from build123d import *

# Parameters (mm, degrees)
CROQUIS1_R              = 25
SALIENTE_EXTRUIR1_DEPTH = 50
CORTAR_EXTRUIR1_REACH   = 102
CROQUIS2_W              = 40
CROQUIS2_H              = 100
CROQUIS3_R              = 25
SALIENTE_EXTRUIR2_DEPTH = 20


with BuildPart() as part:
    # Croquis1 → Saliente-Extruir1 (new body, symmetric)
    with BuildSketch(Plane.XY):
        with BuildLine():
            Line((-50, 0), (50, 0))
            Line((50, 0), (50, 100))
            ThreePointArc((50, 100), (0, 150), (-50, 100))
            Line((-50, 100), (-50, 0))
        make_face()
        with Locations((0, 100)):
            Circle(CROQUIS1_R, mode=Mode.SUBTRACT)
    extrude(amount=SALIENTE_EXTRUIR1_DEPTH, both=True)

    # Croquis2 → Cortar-Extruir1 (cut, up to next)
    with BuildSketch(Plane(origin=(50, 0, 0), x_dir=(0, 0, -1), z_dir=(1, 0, 0)), mode=Mode.PRIVATE) as cortar_extruir1_sk1:
        with Locations((0, 100)):
            Rectangle(CROQUIS2_W, CROQUIS2_H)
    cortar_extruir1_tool1 = extrude(cortar_extruir1_sk1.sketch, amount=-CORTAR_EXTRUIR1_REACH, mode=Mode.PRIVATE) & part.part
    add(cortar_extruir1_tool1.solids().sort_by_distance((50, 100, 0))[0], mode=Mode.SUBTRACT)

    # Croquis3 → Saliente-Extruir2 (add, symmetric)
    with BuildSketch(Plane(origin=(0, 0, 0), x_dir=(0, 0, -1), z_dir=(1, 0, 0))):
        with BuildLine():
            Line((-50, 0), (-50, -150))
            ThreePointArc((-50, -150), (0, -200), (50, -150))
            Line((50, -150), (50, 0))
            Line((50, 0), (-50, 0))
        make_face()
        with Locations((0, -150)):
            Circle(CROQUIS3_R, mode=Mode.SUBTRACT)
    extrude(amount=SALIENTE_EXTRUIR2_DEPTH, both=True)


solid = part.part
Geometry check sheet. Reference: the model listing, model coordinates, mm. A direction names the side the tool comes from. Give positions to 0.01 mm unless a question says otherwise; leave off trailing zeros. Order: outer loops, then holes, each group sorted by start corner. A loop starts at its lowest first (then second) coordinate and runs counter-clockwise, first axis right, second up.
1. Scan lines: line 1 (X direction, y = 100, z = -35); line 2 (X direction, y = -62.5, z = -27); line 3 (Y direction, x = 0, z = -34). Record each from-to range of solid material in increasing order.
Completed:
line 1: x = -50 to -25, 25 to 50
line 2: x = -20 to 20
line 3: y = -186.66 to 75, 125 to 150
2. Sectioned sample at B-B (z = 3). Record the boundary of the cut face in (x, y), then the cut area to 3 significant figures.
Completed:
outline: (-50, 0) - (-20, 0) - (-20, -125.18) - (20, -125.18) - (20, 0) - (50, 0) - (50, 50) - (-50, 50) - close; (-20, -199.91) - (20, -199.91) - (20, -174.82) - (-20, -174.82) - close
area: 11,000 mm2
3. Depth check by flat-ended pin: pin 1 (10 mm diameter, centred on y = -120.5, z = -5, fed in from -X); pin 2 (12 mm diameter, centred on x = -15.5, y = 100, fed in from -Z); pin 3 (12 mm diameter, centred on x = -6, z = -0.5, fed in from +Y); pin 4 (2 mm diameter, centred on x = 9, z = 19.5, fed in from -Y). Enter the tip coordinate at first touch or a pass-through.
Completed:
pin 1: stops at x = -20
pin 2: passes through
pin 3: stops at y = 50
pin 4: stops at y = -196.45
4. Draft check along Y on faces 5 (the face through (-0.28, -128.92, -13.44)), 6 (the face through (12, 77, 20)), 7 (the face through (1.099, 149.988, 35.21)), 8 (the face through (0.28, -199.988, 1.099)). Enter one of: pulls with the +Y half, pulls with the -Y half, needs draft (parallel to the pull), parting line crosses it, or undercut.
Completed:
face 5: undercut
face 6: needs draft
face 7: pulls with the +Y half
face 8: pulls with the -Y half
5. Access from +Z, -Z, +X, -X, +Y, -Y to the whole of each face (thin tool, end or side, straight path). Record for faces 1 (the face through (-50, 40, 1)), 2 (the face through (-35, 0, 1)), 3 (the face through (20, -99, 1)), 4 (the face through (12, 77, -20)).
Completed:
face 1: +Z, -Z, -X, +Y, -Y
face 2: +Z, -Z, -X, -Y
face 3: +Z, -Z, +X, -Y
face 4: +X, -X, +Y
6. Sectioned sample at A-A (x = -13.5). Record the boundary of the cut face in (y, z).
Completed:
outline: (-150, -50) - (78.96, -50) - (78.96, -20) - (50, -20) - (50, 20) - (78.96, 20) - (78.96, 50) - (-150, 50) arc R50 ccw to start; (121.04, -50) - (148.14, -50) - (148.14, -20) - (121.04, -20) - close; (121.04, 20) - (148.14, 20) - (148.14, 50) - (121.04, 50) - close; hole circle Ø50 at (-150, 0)
7. Sectioned sample at C-C (x = 2). Record the boundary of the cut face in (y, z).
Completed:
outline: (-150, -50) - (75.08, -50) - (75.08, -20) - (50, -20) - (50, 20) - (75.08, 20) - (75.08, 50) - (-150, 50) arc R50 ccw to start; (124.92, -50) - (149.96, -50) - (149.96, -20) - (124.92, -20) - close; (124.92, 20) - (149.96, 20) - (149.96, 50) - (124.92, 50) - close; hole circle Ø50 at (-150, 0)
8. Sectioned sample at D-D (y = 118). Record the boundary of the cut face in (x, z), then the cut area to 3 significant figures.
Completed:
outline: (-46.65, -50) - (-17.35, -50) - (-17.35, -20) - (-46.65, -20) - close; (-46.65, 20) - (-17.35, 20) - (-17.35, 50) - (-46.65, 50) - close; (17.35, -50) - (46.65, -50) - (46.65, -20) - (17.35, -20) - close; (17.35, 20) - (46.65, 20) - (46.65, 50) - (17.35, 50) - close
area: 3,520 mm2
